from build123d import *

# Parameters (mm, degrees)
SKETCH1_W           = 436
SKETCH1_H           = 238
BOSS_EXTRUDE1_DEPTH = 6
SKETCH2_W           = 6
SKETCH2_H           = 12
SKETCH2_W_2         = 10
SKETCH2_H_2         = 6
CUT_EXTRUDE1_DEPTH  = 6
SKETCH3_W           = 6
SKETCH3_H           = 34
BOSS_EXTRUDE2_DEPTH = 6
SKETCH4_W           = 39.636363636
SKETCH4_H           = 6
SKETCH4_W_2         = 6
SKETCH4_W_3         = 39.636363637
BOSS_EXTRUDE3_DEPTH = 6
SKETCH5_W           = 60
SKETCH5_H           = 12
SKETCH5_W_2         = 448
SKETCH5_H_2         = 8
BOSS_EXTRUDE4_DEPTH = 6
FILLET1_R           = 20
SKETCH6_W           = 6
SKETCH6_H           = 264
BOSS_EXTRUDE5_DEPTH = 8
SKETCH7_W           = 6
SKETCH7_H           = 12
CUT_EXTRUDE2_DEPTH  = 274.651237892


with BuildPart() as part:
    # Sketch1 → Boss-Extrude1 (new body)
    with BuildSketch(Plane.XY):
        Rectangle(SKETCH1_W, SKETCH1_H)
    extrude(amount=BOSS_EXTRUDE1_DEPTH)

    # Sketch2 → Cut-Extrude1 (cut)
    with BuildSketch(Plane(origin=(0, 0, 0), x_dir=(-1, 0, 0), z_dir=(0, 0, -1))):
        with Locations((191, 86)):
            Rectangle(SKETCH2_W, SKETCH2_H)
        with Locations((191, 14.5)):
            Rectangle(SKETCH2_W, SKETCH2_H)
        with Locations((191, -57)):
            Rectangle(SKETCH2_W, SKETCH2_H)
        with Locations((193, -86)):
            Rectangle(SKETCH2_W_2, SKETCH2_H_2)
    extrude(amount=-CUT_EXTRUDE1_DEPTH, mode=Mode.SUBTRACT)

    # Sketch3 → Boss-Extrude2 (add)
    with BuildSketch(Plane.ZY.offset(218)):
        with Locations((3, 102)):
            Rectangle(SKETCH3_W, SKETCH3_H)
        with Locations((3, 34)):
            Rectangle(SKETCH3_W, SKETCH3_H)
        with Locations((3, -34)):
            Rectangle(SKETCH3_W, SKETCH3_H)
        with Locations((3, -102)):
            Rectangle(SKETCH3_W, SKETCH3_H)
    boss_extrude2 = extrude(amount=BOSS_EXTRUDE2_DEPTH)

    # Mirror1: Boss-Extrude2 across plane
    add(boss_extrude2.mirror(Plane(origin=(0, 0, 0), x_dir=(0, 0, 1), z_dir=(1, 0, 0))))

    # Sketch4 → Boss-Extrude3 (add)
    with BuildSketch(Plane.XZ.offset(119)):
        with Locations((-198.181818182, 3)):
            Rectangle(SKETCH4_W, SKETCH4_H)
        with Locations((-221, 3)):
            Rectangle(SKETCH4_W_2, SKETCH4_H)
        with Locations((-118.909090909, 3)):
            Rectangle(SKETCH4_W, SKETCH4_H)
        with Locations((-39.636363637, 3)):
            Rectangle(SKETCH4_W_3, SKETCH4_H)
        with Locations((39.636363637, 3)):
            Rectangle(SKETCH4_W_3, SKETCH4_H)
        with Locations((118.909090909, 3)):
            Rectangle(SKETCH4_W, SKETCH4_H)
        with Locations((198.181818182, 3)):
            Rectangle(SKETCH4_W, SKETCH4_H)
        with Locations((221, 3)):
            Rectangle(SKETCH4_W_2, SKETCH4_H)
    extrude(amount=BOSS_EXTRUDE3_DEPTH)

    # Sketch5 → Boss-Extrude4 (add)
    with BuildSketch(Plane(origin=(0, 0, 0), x_dir=(-1, 0, 0), z_dir=(0, 0, -1))):
        with Locations((194, -139)):
            Rectangle(SKETCH5_W, SKETCH5_H)
        with Locations((-194, -139)):
            Rectangle(SKETCH5_W, SKETCH5_H)
        with Locations((0, -129)):
            Rectangle(SKETCH5_W_2, SKETCH5_H_2)
    extrude(amount=-BOSS_EXTRUDE4_DEPTH)

    # Fillet1
    # the kernel refuses this fillet: 20 mm, written as the material it adds along each edge
    with BuildSketch(Plane(origin=(164, -133, 0), x_dir=(0, -1, 0), z_dir=(0, 0, 1))) as fillet1_piece_1:
        with BuildLine():
            CenterArc((20, -18.33030278), FILLET1_R, 113.578178478, 66.421821522)
            Line((0, -18.33030278), (-0.4, -18.33030278))
            Line((-0.4, -18.33030278), (-0.4, 0))
            Line((-0.4, 0), (0, 0.4))
            ThreePointArc((0, 0.4), (6, 0.4), (11.84, 0.366606056))
            Line((11.84, 0.366606056), (12, 0))
        make_face()
    extrude(amount=6)
    with BuildSketch(Plane(origin=(-164, -133, 0), x_dir=(1, 0, 0), z_dir=(0, 0, 1))) as fillet1_piece_2:
        with BuildLine():
            CenterArc((18.33030278, -20), FILLET1_R, 90, 66.421821522)
            Line((0, -12), (-0.366606056, -11.84))
            ThreePointArc((-0.366606056, -11.84), (-0.4, -6), (-0.4, 0))
            Line((-0.4, 0), (0, 0.4))
            Line((0, 0.4), (18.33030278, 0.4))
            Line((18.33030278, 0.4), (18.33030278, 0))
        make_face()
    extrude(amount=6)

    # Sketch6 → Boss-Extrude5 (add)
    with BuildSketch(Plane.ZY.offset(224)):
        with Locations((3, -13)):
            Rectangle(SKETCH6_W, SKETCH6_H)
    boss_extrude5 = extrude(amount=BOSS_EXTRUDE5_DEPTH)

    # Mirror2: Boss-Extrude5 across plane
    add(boss_extrude5.mirror(Plane(origin=(0, 0, 0), x_dir=(0, 0, 1), z_dir=(1, 0, 0))))

    # Sketch7 → Cut-Extrude2 (cut, through all)
    with BuildSketch(Plane(origin=(0, 0, 0), x_dir=(-1, 0, 0), z_dir=(0, 0, -1))):
        with Locations((-191, 86)):
            Rectangle(SKETCH7_W, SKETCH7_H)
        with Locations((-191, -3.5)):
            Rectangle(SKETCH7_W, SKETCH7_H)
        with Locations((-191, -93)):
            Rectangle(SKETCH7_W, SKETCH7_H)
    extrude(amount=-CUT_EXTRUDE2_DEPTH, mode=Mode.SUBTRACT)


solid = part.part
CAD build for the part. Positions are in the model's coordinates, mm. A direction names the side the tool comes from. Round coordinates to 2 decimals unless told otherwise and drop trailing zeros. Order: outer loops, then holes, each group sorted by start corner. A loop starts at its lowest first (then second) coordinate and runs counter-clockwise, first axis right, second up. Notation, with made-up numbers: (81.5, 65) -> (112.5, 65) arc R20 cw to (112.5, 85) -> close; hole circle Ø11 at (60.25, 60.25). An arc over 180 degrees is marked (long way). Write item = value, one per line. Start each with the question number.
(1) Cut at B-B, the plane x = -75.5. List the corners of the cut face in (y, z).
(2) Pull direction X, two halves, no side cores. Call faces 3 (the cylindrical face through (156.76, -136.356, 2.958)), 4 (the flat face through (-3, -15, 6)): released by +X, released by -X, zero draft, split by the parting line, or undercut.
(3) Cut at A-A, the plane y = -73. List the corners of the cut face in (x, z), then the cut area to 3 significant figures.
(4) Probe line 1 (X direction, y = -124, z = 2.15); line 2 (X direction, y = 11, z = 5.7); line 3 (X direction, y = 55, z = 2.15). List the from-to ranges inside material, lowest first. Write a range as [from, to].
(5) Cut at D-D, the plane x = 46. List the corners of the cut face in (y, z), then the cut area to 3 significant figures.
(6) Cut at C-C, the plane z = 3.5. State how many separate pieces and enclosed holes the cut face has, then the cut area to 3 significant figures.
(7) Which spindle directions (+Z, -Z, +X, -X, +Y, -Y) get a long thin tool onto all of the face, cutting with end or side? Do faces 1 (the flat face through (-3, -15, 0)), 2 (the cylindrical face through (-156.49, -136.18, 2.96)). Say none if no direction does.
Model answer:
q1.outline = (-133, 0) -> (-125, 0) -> (-125, 6) -> (-133, 6) -> close; (-119, 0) -> (119, 0) -> (119, 6) -> (-119, 6) -> close
q2.face_3 = undercut
q2.face_4 = zero draft
q3.outline = (-232, 0) -> (-224, 0) -> (-224, 6) -> (-232, 6) -> close; (-218, 0) -> (218, 0) -> (218, 6) -> (-218, 6) -> close; (224, 0) -> (232, 0) -> (232, 6) -> (224, 6) -> close
q3.area = 2,710 mm2
q4.line_1 = [-232, -178.36], [-138.73, -99.09], [-59.45, -19.82], [19.82, 59.45], [99.09, 138.73], [178.36, 232]
q4.line_2 = [-232, -224], [-218, -194], [-188, 218], [224, 232]
q4.line_3 = [-232, -224], [-218, 218], [224, 232]
q5.outline = (-133, 0) -> (119, 0) -> (119, 6) -> (-133, 6) -> close
q5.area = 1,510 mm2
q6.separate_pieces = 1
q6.enclosed_holes = 18
q6.area = 116,000 mm2
q7.face_1 = -Z, +X, -X, +Y, -Y
q7.face_2 = +Z, -Z, -Y
